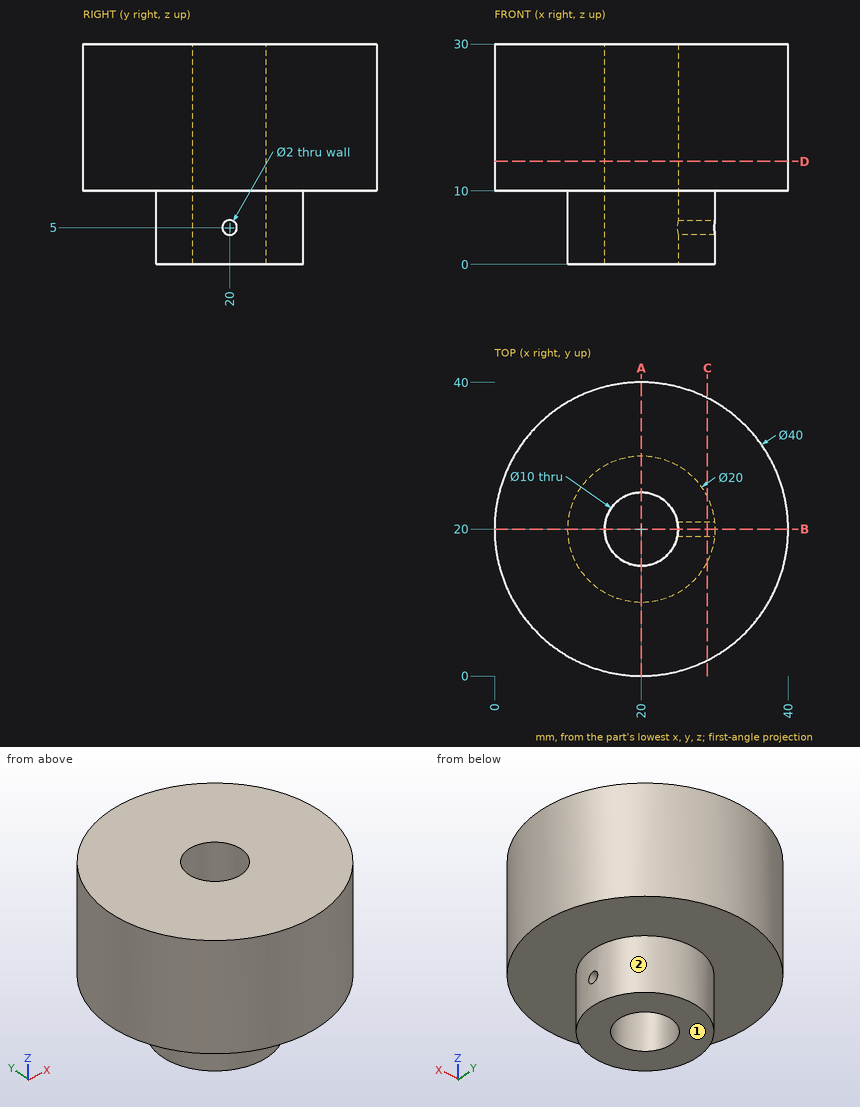
Print and shaded views of the part. All mm, measured from the part's lowest x, y and z. A direction names the side the tool comes from. Give positions to 0.01 mm unless a question says otherwise; leave off trailing zeros. Loops run counter-clockwise (first coordinate to the right, second up) from the corner with the lowest first, then second, coordinate; pieces in that order, holes last. Notation, with made-up numbers: (-39, -17) -> (10, -17) arc R17 cw to (10, 8) -> close; hole circle Ø10 at (-23.5, 67). An arc over 180 degrees is marked (long way). Use CSV: the item, a comma, the result in double quotes. Start each with the question number.
1) Slice it at D-D on z = 14. Give the cut face in (x, y), plus the area to 3 significant figures.
2) Tool access for the marked faces 1 and 2: list every direction of +Z, -Z, +X, -X, +Y, -Y with a clear straight run to the whole face (end or side of a thin tool).
3) Slice it at B-B on y = 20. Give the cut face in (x, z).
4) Slice it at A-A on x = 20. Give the cut face in (y, z).
5) Wall check: line 1 (Z direction, x = 27.85, y = 20); line 2 (Z direction, x = 7, y = 21.5); line 3 (Y direction, x = 20.5, z = 2). Give the ranges that are in metal, low to high.
6) Flat gauge pins, fed straight in: pin 1 Ø1 at (y, z) = (9.5, 11.5) entering from +X; pin 2 Ø10 at (x, z) = (19.5, 21) entering from -Y; pin 3 Ø10 at (x, z) = (27, 21.5) entering from +Y; pin 4 Ø6 at (x, y) = (20, 20) entering from +Z. Where does each tip first touch, or does it go through?
7) Slice it at C-C on x = 29. Give the cut face in (y, z), plus the area to 3 significant figures.
Computed values:
1,outline,"circle Ø40 at (20, 20); hole circle Ø10 at (20, 20)"
1,area,"1,180 mm^2"
2,face 1,"-Z, +X, -X, +Y, -Y"
2,face 2,"-Z"
3,outline,"(0, 10) -> (10, 10) -> (10, 0) -> (15, 0) -> (15, 30) -> (0, 30) -> close; (25, 0) -> (30, 0) -> (30, 4) -> (25, 4) -> close; (25, 6) -> (30, 6) -> (30, 10) -> (40, 10) -> (40, 30) -> (25, 30) -> close"
4,outline,"(0, 10) -> (10, 10) -> (10, 0) -> (15, 0) -> (15, 30) -> (0, 30) -> close; (25, 0) -> (30, 0) -> (30, 10) -> (40, 10) -> (40, 30) -> (25, 30) -> close"
5,line 1,"z = 0 to 4, 6 to 30"
5,line 2,"z = 10 to 30"
5,line 3,"y = 10.01 to 15.03, 24.97 to 29.99"
6,pin 1,"stops at x = 37.32"
6,pin 2,"stops at y = 0"
6,pin 3,"stops at y = 39.9"
6,pin 4,"passes through"
7,outline,"(2.14, 10) -> (15.64, 10) -> (15.64, 0) -> (24.36, 0) -> (24.36, 10) -> (37.86, 10) -> (37.86, 30) -> (2.14, 30) -> close; hole circle Ø2 at (20, 5)"
7,area,"798 mm^2"
